Work out the finished part from the listing and answer in its coordinate system (mm). Face numbers are marked on the shaded views. A direction names the side the tool comes from. Give positions to 0.01 mm unless a question says otherwise; leave off trailing zeros. Write each loop counter-clockwise with the first axis right and the second up, starting at its lowest first coordinate (ties: lowest second). Pieces come first, ordered by that corner, then holes. Notation, with made-up numbers: (-35.75, 82) -> (21.25, 82) arc R19 ccw to (21.25, 119) -> close; hole circle Ø10 at (64.25, 29). An arc over 180 degrees is marked (long way). Write item = value, one per line. Start each with the question number.
from build123d import *

# Parameters (mm, degrees)
ESTRUSIONE_ESTRUSIONE1_DEPTH  = 12
ESTRUSIONE_ESTRUSIONE2_START  = -1.85
ESTRUSIONE_ESTRUSIONE2_DEPTH  = 1.85
ESTRUSIONE_ESTRUSIONE3_DEPTH  = 1.85
ESTRUSIONE_ESTRUSIONE4_DEPTH  = 23.5
ESTRUSIONE_ESTRUSIONE5_START  = 1.85
ESTRUSIONE_ESTRUSIONE5_DEPTH  = 1.85
ESTRUSIONE_ESTRUSIONE6_START  = 8.3
ESTRUSIONE_ESTRUSIONE6_DEPTH  = 8.3
ESTRUSIONE_ESTRUSIONE7_START  = 1.85
ESTRUSIONE_ESTRUSIONE7_DEPTH  = 1.85
ESTRUSIONE_ESTRUSIONE8_DEPTH  = 23.5
ESTRUSIONE_ESTRUSIONE9_START  = 1.85
ESTRUSIONE_ESTRUSIONE9_DEPTH  = 1.85
ESTRUSIONE_ESTRUSIONE10_START = 8.3
ESTRUSIONE_ESTRUSIONE10_DEPTH = 8.3
ESTRUSIONE_ESTRUSIONE11_START = 1.85
ESTRUSIONE_ESTRUSIONE11_DEPTH = 1.85
SCHIZZO12_R                   = 2.25
TAGLIO_ESTRUSIONE1_DEPTH      = 95.695564838
SCHIZZO13_R                   = 2.1
TAGLIO_ESTRUSIONE2_DEPTH      = 6
SCHIZZO15_R                   = 2.1
TAGLIO_ESTRUSIONE4_DEPTH      = 5
SCHIZZO16_R                   = 3.75
TAGLIO_ESTRUSIONE5_DEPTH      = 2


with BuildPart() as part:
    # Schizzo1 → Estrusione-Estrusione1 (new body)
    with BuildSketch(Plane.XY):
        with BuildLine():
            Line((-12.1, 0), (-21, 0))
            Line((-21, 0), (-21, -17.1))
            Line((-21, -17.1), (21, -17.1))
            Line((21, -17.1), (21, 0))
            Line((21, 0), (12.1, 0))
            ThreePointArc((12.1, 0), (0, -12.1), (-12.1, 0))
        make_face()
        Polygon((-42, -46.5), (-42, -54.5), (42, -54.5), (42, -46.5), (32, -46.5), (23.95754717, 0), (21, 0), (21, -17.1), (-21, -17.1), (-21, 0), (-23.95754717, 0), (-32, -46.5), align=None)
    extrude(amount=ESTRUSIONE_ESTRUSIONE1_DEPTH)

    # Schizzo2 → Estrusione-Estrusione2 (add)
    with BuildSketch(Plane.XY.offset(12).offset(ESTRUSIONE_ESTRUSIONE2_START)):
        with BuildLine():
            Line((12.1, 0), (10.5, 0))
            ThreePointArc((10.5, 0), (0, -10.5), (-10.5, 0))
            Line((-10.5, 0), (-12.1, 0))
            ThreePointArc((-12.1, 0), (0, -12.1), (12.1, 0))
        make_face()
    extrude(amount=ESTRUSIONE_ESTRUSIONE2_DEPTH)

    # Schizzo3 → Estrusione-Estrusione3 (add)
    with BuildSketch(Plane(origin=(0, 0, 0), x_dir=(-1, 0, 0), z_dir=(0, 0, -1))):
        with BuildLine():
            Line((12.1, 0), (10.5, 0))
            ThreePointArc((10.5, 0), (0, -10.5), (-10.5, 0))
            Line((-10.5, 0), (-12.1, 0))
            ThreePointArc((-12.1, 0), (0, -12.1), (12.1, 0))
        make_face()
    extrude(amount=-ESTRUSIONE_ESTRUSIONE3_DEPTH)

    # Schizzo4 → Estrusione-Estrusione4 (add)
    with BuildSketch(Plane(origin=(0, 0, 0), x_dir=(-1, 0, 0), z_dir=(0, 0, -1))):
        with BuildLine():
            Line((-27.454507827, -46.5), (-32, -46.5))
            Line((-32, -46.5), (-42, -46.5))
            Line((-42, -46.5), (-42, -54.5))
            Line((-42, -54.5), (42, -54.5))
            Line((42, -54.5), (42, -46.5))
            Line((42, -46.5), (32, -46.5))
            Line((32, -46.5), (27.454507827, -46.5))
            ThreePointArc((27.454507827, -46.5), (0, -54), (-27.454507827, -46.5))
        make_face()
    extrude(amount=ESTRUSIONE_ESTRUSIONE4_DEPTH)

    # Schizzo5 → Estrusione-Estrusione5 (add)
    with BuildSketch(Plane(origin=(0, 0, -23.5), x_dir=(-1, 0, 0), z_dir=(0, 0, -1)).offset(ESTRUSIONE_ESTRUSIONE5_START)):
        with BuildLine():
            Line((23.95754717, 0), (10.5, 0))
            ThreePointArc((10.5, 0), (0, -10.5), (-10.5, 0))
            Line((-10.5, 0), (-23.95754717, 0))
            Line((-23.95754717, 0), (-32, -46.5))
            Line((-32, -46.5), (-42, -46.5))
            Line((-42, -46.5), (-42, -54.5))
            Line((-42, -54.5), (42, -54.5))
            Line((42, -54.5), (42, -46.5))
            Line((42, -46.5), (32, -46.5))
            Line((32, -46.5), (23.95754717, 0))
        make_face()
    extrude(amount=-ESTRUSIONE_ESTRUSIONE5_DEPTH)

    # Schizzo6 → Estrusione-Estrusione6 (add)
    with BuildSketch(Plane(origin=(0, 0, -25.35), x_dir=(-1, 0, 0), z_dir=(0, 0, -1)).offset(ESTRUSIONE_ESTRUSIONE6_START)):
        with BuildLine():
            ThreePointArc((12.1, 0), (0, -12.1), (-12.1, 0))
            Line((-12.1, 0), (-23.95754717, 0))
            Line((-23.95754717, 0), (-32, -46.5))
            Line((-32, -46.5), (-42, -46.5))
            Line((-42, -46.5), (-42, -54.5))
            Line((-42, -54.5), (42, -54.5))
            Line((42, -54.5), (42, -46.5))
            Line((42, -46.5), (32, -46.5))
            Line((32, -46.5), (23.95754717, 0))
            Line((23.95754717, 0), (12.1, 0))
        make_face()
    extrude(amount=-ESTRUSIONE_ESTRUSIONE6_DEPTH)

    # Schizzo7 → Estrusione-Estrusione7 (add)
    with BuildSketch(Plane(origin=(0, 0, -33.65), x_dir=(-1, 0, 0), z_dir=(0, 0, -1)).offset(ESTRUSIONE_ESTRUSIONE7_START)):
        with BuildLine():
            Line((23.95754717, 0), (10.5, 0))
            ThreePointArc((10.5, 0), (0, -10.5), (-10.5, 0))
            Line((-10.5, 0), (-23.95754717, 0))
            Line((-23.95754717, 0), (-32, -46.5))
            Line((-32, -46.5), (-42, -46.5))
            Line((-42, -46.5), (-42, -54.5))
            Line((-42, -54.5), (42, -54.5))
            Line((42, -54.5), (42, -46.5))
            Line((42, -46.5), (32, -46.5))
            Line((32, -46.5), (23.95754717, 0))
        make_face()
    extrude(amount=-ESTRUSIONE_ESTRUSIONE7_DEPTH)

    # Schizzo8 → Estrusione-Estrusione8 (add)
    with BuildSketch(Plane(origin=(0, 0, -35.5), x_dir=(-1, 0, 0), z_dir=(0, 0, -1))):
        Polygon((-32, -46.5), (32, -46.5), (42, -46.5), (42, -54.5), (-42, -54.5), (-42, -46.5), align=None)
    extrude(amount=ESTRUSIONE_ESTRUSIONE8_DEPTH)

    # Schizzo9 → Estrusione-Estrusione9 (add)
    with BuildSketch(Plane(origin=(0, 0, -59), x_dir=(-1, 0, 0), z_dir=(0, 0, -1)).offset(ESTRUSIONE_ESTRUSIONE9_START)):
        with BuildLine():
            Line((23.95754717, 0), (10.5, 0))
            ThreePointArc((10.5, 0), (0, -10.5), (-10.5, 0))
            Line((-10.5, 0), (-23.95754717, 0))
            Line((-23.95754717, 0), (-32, -46.5))
            Line((-32, -46.5), (-42, -46.5))
            Line((-42, -46.5), (-42, -54.5))
            Line((-42, -54.5), (42, -54.5))
            Line((42, -54.5), (42, -46.5))
            Line((42, -46.5), (32, -46.5))
            Line((32, -46.5), (23.95754717, 0))
        make_face()
    extrude(amount=-ESTRUSIONE_ESTRUSIONE9_DEPTH)

    # Schizzo10 → Estrusione-Estrusione10 (add)
    with BuildSketch(Plane(origin=(0, 0, -60.85), x_dir=(-1, 0, 0), z_dir=(0, 0, -1)).offset(ESTRUSIONE_ESTRUSIONE10_START)):
        with BuildLine():
            ThreePointArc((12.1, 0), (0, -12.1), (-12.1, 0))
            Line((-12.1, 0), (-23.95754717, 0))
            Line((-23.95754717, 0), (-32, -46.5))
            Line((-32, -46.5), (-42, -46.5))
            Line((-42, -46.5), (-42, -54.5))
            Line((-42, -54.5), (42, -54.5))
            Line((42, -54.5), (42, -46.5))
            Line((42, -46.5), (32, -46.5))
            Line((32, -46.5), (23.95754717, 0))
            Line((23.95754717, 0), (12.1, 0))
        make_face()
    extrude(amount=-ESTRUSIONE_ESTRUSIONE10_DEPTH)

    # Schizzo11 → Estrusione-Estrusione11 (add)
    with BuildSketch(Plane(origin=(0, 0, -69.15), x_dir=(-1, 0, 0), z_dir=(0, 0, -1)).offset(ESTRUSIONE_ESTRUSIONE11_START)):
        with BuildLine():
            Line((23.95754717, 0), (10.5, 0))
            ThreePointArc((10.5, 0), (0, -10.5), (-10.5, 0))
            Line((-10.5, 0), (-23.95754717, 0))
            Line((-23.95754717, 0), (-32, -46.5))
            Line((-32, -46.5), (-42, -46.5))
            Line((-42, -46.5), (-42, -54.5))
            Line((-42, -54.5), (42, -54.5))
            Line((42, -54.5), (42, -46.5))
            Line((42, -46.5), (32, -46.5))
            Line((32, -46.5), (23.95754717, 0))
        make_face()
    extrude(amount=-ESTRUSIONE_ESTRUSIONE11_DEPTH)

    # Schizzo12 → Taglio-Estrusione1 (cut, through all)
    with BuildSketch(Plane(origin=(0, -46.5, 0), x_dir=(1, 0, 0), z_dir=(0, 1, 0))):
        with Locations(Location((37, -6.5, 0), (0, 0, 270))):
            Circle(SCHIZZO12_R)
        with Locations(Location((37, 28.5, 0), (0, 0, 270))):
            Circle(SCHIZZO12_R)
        with Locations(Location((37, 65.5, 0), (0, 0, 270))):
            Circle(SCHIZZO12_R)
        with Locations(Location((-37, -6.5, 0), (0, 0, 270))):
            Circle(SCHIZZO12_R)
        with Locations(Location((-37, 28.5, 0), (0, 0, 270))):
            Circle(SCHIZZO12_R)
        with Locations(Location((-37, 65.5, 0), (0, 0, 270))):
            Circle(SCHIZZO12_R)
    extrude(amount=-TAGLIO_ESTRUSIONE1_DEPTH, mode=Mode.SUBTRACT)

    # Schizzo13 → Taglio-Estrusione2 (cut)
    with BuildSketch(Plane(origin=(0, 0, 0), x_dir=(1, 0, 0), z_dir=(0, 1, 0))):
        with Locations(Location((18.028773585, -6, 0), (0, 0, 180))):
            Circle(SCHIZZO13_R)
        with Locations(Location((-18.028773585, -6, 0), (0, 0, 180))):
            Circle(SCHIZZO13_R)
        with Locations(Location((18.028773585, 29.5, 0), (0, 0, 180))):
            Circle(SCHIZZO13_R)
        with Locations(Location((-18.028773585, 29.5, 0), (0, 0, 180))):
            Circle(SCHIZZO13_R)
        with Locations(Location((18.028773585, 65, 0), (0, 0, 180))):
            Circle(SCHIZZO13_R)
        with Locations(Location((-18.028773585, 65, 0), (0, 0, 180))):
            Circle(SCHIZZO13_R)
    extrude(amount=-TAGLIO_ESTRUSIONE2_DEPTH, mode=Mode.SUBTRACT)

    # Schizzo15 → Taglio-Estrusione4 (cut)
    with BuildSketch(Plane(origin=(0, -6, 0), x_dir=(1, 0, 0), z_dir=(0, 1, 0))):
        with Locations(Location((-18.028773585, 65, 0), (0, 0, 180))):
            Circle(SCHIZZO15_R)
        with Locations(Location((18.028773585, 65, 0), (0, 0, 180))):
            Circle(SCHIZZO15_R)
        with Locations(Location((18.028773585, 29.5, 0), (0, 0, 180))):
            Circle(SCHIZZO15_R)
        with Locations(Location((-18.028773585, 29.5, 0), (0, 0, 180))):
            Circle(SCHIZZO15_R)
        with Locations(Location((-18.028773585, -6, 0), (0, 0, 180))):
            Circle(SCHIZZO15_R)
        with Locations(Location((18.028773585, -6, 0), (0, 0, 180))):
            Circle(SCHIZZO15_R)
    extrude(amount=-TAGLIO_ESTRUSIONE4_DEPTH, mode=Mode.SUBTRACT)

    # Schizzo16 → Taglio-Estrusione5 (cut)
    with BuildSketch(Plane(origin=(0, -46.5, 0), x_dir=(1, 0, 0), z_dir=(0, 1, 0))):
        with Locations(Location((37, -6.5, 0), (0, 0, 270))):
            Circle(SCHIZZO16_R)
        with Locations(Location((37, 28.5, 0), (0, 0, 270))):
            Circle(SCHIZZO16_R)
        with Locations(Location((37, 65.5, 0), (0, 0, 270))):
            Circle(SCHIZZO16_R)
        with Locations(Location((-37, 65.5, 0), (0, 0, 270))):
            Circle(SCHIZZO16_R)
        with Locations(Location((-37, 28.5, 0), (0, 0, 270))):
            Circle(SCHIZZO16_R)
        with Locations(Location((-37, -6.5, 0), (0, 0, 270))):
            Circle(SCHIZZO16_R)
    extrude(amount=-TAGLIO_ESTRUSIONE5_DEPTH, mode=Mode.SUBTRACT)


solid = part.part
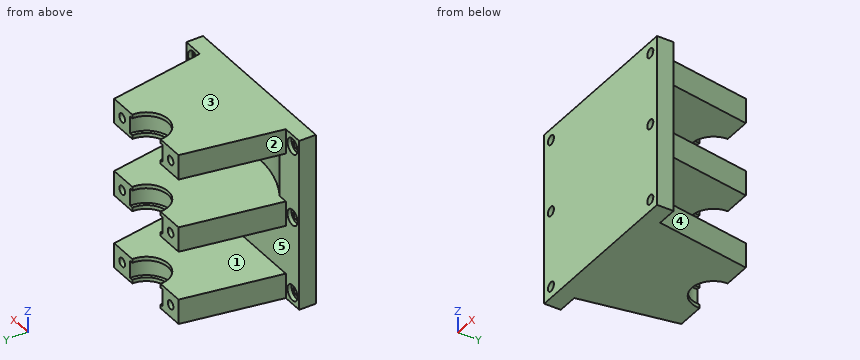
(1) A cutting plane is placed at D-D, the plane z = -65. State how many separate pieces and enclosed holes the cut face has, then the cut area to 3 significant figures.
(2) Determine the mould class of the marked faces 3, 4 and 5 for opening direction Z: pulls with the +Z half, pulls with the -Z half, needs draft (parallel to the pull), parting line crosses it, or undercut.
(3) A cutting plane is placed at C-C, the plane z = -3.5. Write down the section's boundary in (x, y), then the cut area to 3 significant figures.
(4) Find the intervals of material crossed by line 1 along Z through (x, y) = (-0.5, -23); line 2 along X through (y, z) = (-46.95, 6.5); line 3 along X through (y, z) = (-51.85, 6.5), in increasing order.
(5) A cutting plane is placed at B-B, the plane y = -26. Write down the section's boundary in (x, z), then the cut area to 3 significant figures.
(6) Each of these flat-tipped pins is pushed along its axis until it touches: pin 1 (6 mm diameter, centred on y = -12.5, z = -58.5, fed in from -X); pin 2 (4 mm diameter, centred on x = 35.5, z = -28.5, fed in from +Y); pin 3 (8.5 mm diameter, centred on x = -37, z = -65.5, fed in from +Y); pin 4 (4 mm diameter, centred on x = 37, z = -65.5, fed in from -Y). Where does it stop, or does it pass through?
(7) A cutting plane is placed at A-A, the plane x = -37. Write down the section's boundary in (y, z), then the cut area to 3 significant figures.
(8) For the marked faces 1 and 2, determine the directions among +Z, -Z, +X, -X, +Y, -Y from which every point of the face is accessible in a straight line to the end or side of a thin tool.
Results list:
q1.separate_pieces = 3
q1.enclosed_holes = 0
q1.area = 2,870 mm²
q2.face_3 = pulls with the +Z half
q2.face_4 = needs draft
q2.face_5 = undercut
q3.outline = (-42, -54.5) -> (42, -54.5) -> (42, -46.5) -> (27.45, -46.5) arc R54 cw to (-27.45, -46.5) -> (-42, -46.5) -> close
q3.area = 393 mm²
q4.line_1 = -71 to -59, -35.5 to -23.5, 0 to 12
q4.line_2 = -42 to -40.75, -33.25 to 33.25, 40.75 to 42
q4.line_3 = -42 to -39.25, -34.75 to 34.75, 39.25 to 42
q5.outline = (-28.45, -71) -> (28.45, -71) -> (28.45, -59) -> (-28.45, -59) -> close; (-28.45, -35.5) -> (28.45, -35.5) -> (28.45, -23.5) -> (-28.45, -23.5) -> close; (-28.45, 0) -> (28.45, 0) -> (28.45, 12) -> (-28.45, 12) -> close
q5.area = 2,050 mm²
q6.pin_1 = -26.63
q6.pin_2 = -48.5
q6.pin_3 = -46.5
q6.pin_4 = through
q7.outline = (-54.5, -71) -> (-46.5, -71) -> (-46.5, -69.25) -> (-48.5, -69.25) -> (-48.5, -67.75) -> (-54.5, -67.75) -> close; (-54.5, -63.25) -> (-48.5, -63.25) -> (-48.5, -61.75) -> (-46.5, -61.75) -> (-46.5, -32.25) -> (-48.5, -32.25) -> (-48.5, -30.75) -> (-54.5, -30.75) -> close; (-54.5, -26.25) -> (-48.5, -26.25) -> (-48.5, -24.75) -> (-46.5, -24.75) -> (-46.5, 2.75) -> (-48.5, 2.75) -> (-48.5, 4.25) -> (-54.5, 4.25) -> close; (-54.5, 8.75) -> (-48.5, 8.75) -> (-48.5, 10.25) -> (-46.5, 10.25) -> (-46.5, 12) -> (-54.5, 12) -> close
q7.area = 538 mm²
q8.face_1 = +X, -X, +Y
q8.face_2 = +Z, -Z, -X, +Y
